Model file for the job. Use its own axes, mm. Round coordinates to 2 decimals unless told otherwise and drop trailing zeros. Loops run counter-clockwise (first coordinate to the right, second up) from the corner with the lowest first, then second, coordinate; pieces in that order, holes last. Notation, with made-up numbers: M 70,34 L 117,34 A27 cw 117,51 Z; hole C 79.25,-2 d11. An arc over 180 degrees is marked long. Use a Markdown table: item, result. Add a question column.
Item 1: Pin check, flat tips, straight feed: P1, Ø0.9, axis at x = 70, y = 1, coming from the +Z side; P2, Ø6, axis at x = 73.5, z = -9, coming from the +Y side. Stop position of each tip, or through.
Item 2: Saw through at A-A on x = 31. Write the cut outline in (y, z).
Item 3: Wall check: L1, parallel to X at y = 2.8, z = -2.75; L2, parallel to X at y = 1.3, z = -11.5; L3, parallel to Z at x = 84.5, y = 2.8. Give the ranges that are in metal, low to high. Write a range as from..to.
Item 4: Saw through at B-B on x = 3. Write the cut outline in (y, z), then the cut area to 3 significant figures.
Item 5: Saw through at C-C on y = 1.15. Write the cut outline in (x, z).
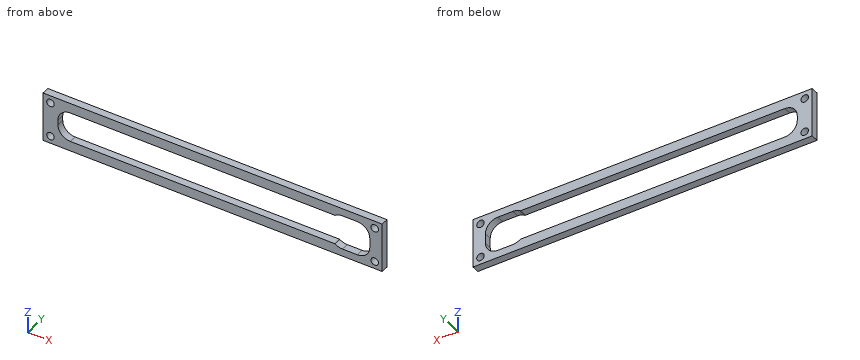
```python
from build123d import *

# Parameters (mm, degrees)
SKETCH1_W           = 136.427821805
SKETCH1_H           = 20
SKETCH1_R           = 1.5
SKETCH1_W_2         = 124.427821805
SKETCH1_H_2         = 12
BOSS_EXTRUDE1_DEPTH = 3
CUT_EXTRUDE1_DEPTH  = 138.918637473
FILLET1_R           = 5


with BuildPart() as part:
    # Sketch1 → Boss-Extrude1 (new body)
    with BuildSketch(Plane(origin=(0, 0, 0), x_dir=(1, 0, 0), z_dir=(0, 1, 0))):
        with Locations((68.213910903, 10)):
            Rectangle(SKETCH1_W, SKETCH1_H)
        with Locations(Location((3, 17, 0), (0, 0, 270))):
            Circle(SKETCH1_R, mode=Mode.SUBTRACT)
        with Locations(Location((3, 3, 0), (0, 0, 90))):
            Circle(SKETCH1_R, mode=Mode.SUBTRACT)
        with Locations(Location((133.427821805, 3, 0), (0, 0, 270))):
            Circle(SKETCH1_R, mode=Mode.SUBTRACT)
        with Locations(Location((133.427821805, 17, 0), (0, 0, 90))):
            Circle(SKETCH1_R, mode=Mode.SUBTRACT)
        with Locations((68.213910903, 10)):
            Rectangle(SKETCH1_W_2, SKETCH1_H_2, mode=Mode.SUBTRACT)
    extrude(amount=BOSS_EXTRUDE1_DEPTH)

    # Sketch2 → Cut-Extrude1 (cut, through all)
    with BuildSketch(Plane(origin=(0, 3, 0), x_dir=(1, 0, 0), z_dir=(0, 1, 0))):
        Polygon((117.427821805, 17), (117.427821805, 16), (130.427821805, 16), (130.427821805, 4), (117.427821805, 4), (117.427821805, 3), (131.427821805, 3), (131.427821805, 17), align=None)
    extrude(amount=-CUT_EXTRUDE1_DEPTH, mode=Mode.SUBTRACT)

    # Fillet1
    # the kernel refuses this fillet: 5 mm, written as the material it adds along each edge
    with BuildSketch(Plane(origin=(131.427821805, 3, -17), x_dir=(0, 0, 1), z_dir=(0, -1, 0)), Plane(origin=(131.427821805, 3, -3), x_dir=(-1, 0, 0), z_dir=(0, -1, 0)), Plane(origin=(6, 0, -16), x_dir=(0, 0, 1), z_dir=(0, 1, 0))) as fillet1_piece_1:
        with BuildLine():
            CenterArc((FILLET1_R, FILLET1_R), FILLET1_R, 180, 90)
            Line((0, FILLET1_R), (-FILLET1_R * 0.02, FILLET1_R))
            Line((-FILLET1_R * 0.02, FILLET1_R), (-FILLET1_R * 0.02, -FILLET1_R * 0.02))
            Line((-FILLET1_R * 0.02, -FILLET1_R * 0.02), (FILLET1_R, -FILLET1_R * 0.02))
            Line((FILLET1_R, -FILLET1_R * 0.02), (FILLET1_R, 0))
        make_face()
    extrude(amount=3)
    with BuildSketch(Plane(origin=(117.427821805, 3, -17), x_dir=(1, 0, 0), z_dir=(0, -1, 0))) as fillet1_piece_2:
        with BuildLine():
            CenterArc((3, 5), FILLET1_R, 233.130102354, 36.869897646)
            Line((0, 1), (-0.06, 0.92))
            ThreePointArc((-0.06, 0.92), (-0.1, 0.5), (-0.1, 0))
            Line((-0.1, 0), (0, -0.1))
            Line((0, -0.1), (3, -0.1))
            Line((3, -0.1), (3, 0))
        make_face()
    extrude(amount=3)
    with BuildSketch(Plane(origin=(117.427821805, 3, -3), x_dir=(0, 0, -1), z_dir=(0, -1, 0))) as fillet1_piece_3:
        with BuildLine():
            CenterArc((5, 3), FILLET1_R, 180, 36.869897646)
            Line((0, 3), (-0.1, 3))
            Line((-0.1, 3), (-0.1, 0))
            Line((-0.1, 0), (0, -0.1))
            ThreePointArc((0, -0.1), (0.5, -0.1), (0.92, -0.06))
            Line((0.92, -0.06), (1, 0))
        make_face()
    extrude(amount=3)
    with BuildSketch(Plane(origin=(6, 0, -4), x_dir=(0, 0, -1), z_dir=(0, 1, 0))) as fillet1_piece_4:
        with BuildLine():
            CenterArc((FILLET1_R, -FILLET1_R), FILLET1_R, 90, 90)
            Line((0, -FILLET1_R), (-FILLET1_R * 0.02, -FILLET1_R))
            Line((-FILLET1_R * 0.02, -FILLET1_R), (-FILLET1_R * 0.02, FILLET1_R * 0.02))
            Line((-FILLET1_R * 0.02, FILLET1_R * 0.02), (FILLET1_R, FILLET1_R * 0.02))
            Line((FILLET1_R, FILLET1_R * 0.02), (FILLET1_R, 0))
        make_face()
    extrude(amount=3)


solid = part.part
```
Entries:
| question | item | result |
|---|---|---|
| 1 | P1 | z = 0 |
| 1 | P2 | through |
| 2 | outline | M 0,-20 L 3,-20 L 3,-16 L 0,-16 Z; M 0,-4 L 3,-4 L 3,0 L 0,0 Z |
| 3 | L1 | 0..1.52, 4.48..131.95, 134.91..136.43 |
| 3 | L2 | 0..6.03, 131.43..136.43 |
| 3 | L3 | -20..-16, -4..0 |
| 4 | outline | M 0,-20 L 3,-20 L 3,-18.5 L 0,-18.5 Z; M 0,-15.5 L 3,-15.5 L 3,-4.5 L 0,-4.5 Z; M 0,-1.5 L 3,-1.5 L 3,0 L 0,0 Z |
| 4 | area | 42.0 mm2 |
| 5 | outline | M 0,-20 L 136.43,-20 L 136.43,0 L 0,0 Z; hole C 3,-17 d3; hole C 3,-3 d3; hole M 6,-11 A5 ccw 11,-16 L 117.43,-16 A5 ccw 120.43,-17 L 126.43,-17 A5 ccw 131.43,-12 L 131.43,-8 A5 ccw 126.43,-3 L 120.43,-3 A5 ccw 117.43,-4 L 11,-4 A5 ccw 6,-9 Z; hole C 133.43,-17 d3; hole C 133.43,-3 d3 |
